The model under review builds one solid part; all positions refer to its coordinate system, in mm. Coordinates: 2 decimals unless noted, no trailing zeros. Order: outer loops, then holes, each group sorted by start corner. A loop starts at its lowest first (then second) coordinate and runs counter-clockwise, first axis right, second up. Notation, with made-up numbers: (25, -39) -> (77, -39) arc R34 cw to (77, -4) -> close; hole circle Ø5 at (-32, 73). An arc over 180 degrees is marked (long way). Use one line per item in the form item = value. Start each with the question number.
(1) Wall thickness on line 1 along Y through (x, z) = (-6.75, -257); line 2 along Y through (x, z) = (-4.25, -515); line 3 along Y through (x, z) = (-3, -60): over which ranges is each line inside the solid? List them lowest first.
(2) Insertion check: pin 1 Ø6 at (y, z) = (47, -1044.5) entering from +X (3 decimals); pin 2 Ø1.1 at (y, z) = (113.5, -835) entering from +X; pin 3 Ø5 at (x, z) = (-8.5, -517) entering from +Y. Each pin has a flat end and moves straight along its axis. Give the tip position at first contact, or say it passes through.
(3) Take a section at A-A (y = 32.5). State the section outline as (x, z) points (3 decimals), then the cut area to 3 significant figures.
(4) Mouldability with a two-part tool opening along Y and no side actions: class faces 1 (the flat face through (-8.255, 56, -618)), 2 (the flat face through (-9.525, 55, -618)) as +Y half, -Y half, draft (parallel to the pull), parting line (faces both ways), or undercut.
```python
from build123d import *

# Parameters (mm, degrees)
EXTRUDE_THIN1_DEPTH = 1254.125
FILLET1_R           = 1.27


with BuildPart() as part:
    # Sketch1 → Extrude-Thin1 (new body)
    with BuildSketch(Plane.XY):
        with BuildLine():
            Line((0, 0), (-9.525, 0))
            Line((-9.525, 0), (-9.525, 109.5375))
            ThreePointArc((-9.525, 109.5375), (-8.59506403, 111.78256403), (-6.35, 112.7125))
            Line((-6.35, 112.7125), (-6.35, 115.8875))
            ThreePointArc((-6.35, 115.8875), (-3.884748595, 117.779153935), (-5.073891971, 120.65))
            ThreePointArc((-5.073891971, 120.65), (-6.263035347, 123.520846065), (-3.797783942, 125.4125))
            Line((-3.797783942, 125.4125), (0, 125.4125))
            Line((0, 125.4125), (0, 124.1425))
            Line((0, 124.1425), (-3.797783942, 124.1425))
            ThreePointArc((-3.797783942, 124.1425), (-5.036309547, 123.192145878), (-4.438891971, 121.749852263))
            ThreePointArc((-4.438891971, 121.749852263), (-2.544105078, 118.08687128), (-5.08, 114.834659111))
            Line((-5.08, 114.834659111), (-5.08, 110.957403166))
            ThreePointArc((-5.08, 110.957403166), (-7.127712993, 111.27651912), (-8.255, 109.5375))
            Line((-8.255, 109.5375), (-8.255, 1.27))
            Line((-8.255, 1.27), (0, 1.27))
            Line((0, 1.27), (0, 0))
        make_face()
    extrude(amount=-EXTRUDE_THIN1_DEPTH)

    # Fillet1
    fillet1_edges = [part.edges().sort_by_distance(p)[0] for p in [
        (-5.08, 110.957403166, -627.0625),
        (-9.525, 0, -627.0625),
        (-6.35, 115.8875, -627.0625),
    ]]
    fillet(fillet1_edges, radius=FILLET1_R)


solid = part.part
```
Findings:
q1.line_1 = 0 to 1.27, 111.4 to 112.69
q1.line_2 = 0 to 1.27, 115.25 to 116.99, 119.89 to 121.63, 124.06 to 125.37
q1.line_3 = 0 to 1.27, 116.6 to 120.28, 124.14 to 125.41
q2.pin_1 = -8.255
q2.pin_2 = -5.08
q2.pin_3 = 124.15
q3.outline = (-9.525, -1254.125) -> (-8.255, -1254.125) -> (-8.255, 0) -> (-9.525, 0) -> close
q3.area = 1,590 mm²
q4.face_1 = undercut
q4.face_2 = draft
